Check sheet for the modelled part. Datum: model origin and axes. Units: mm. Round coordinates to 2 decimals unless told otherwise and drop trailing zeros. Write each loop counter-clockwise with the first axis right and the second up, starting at its lowest first coordinate (ties: lowest second). Pieces come first, ordered by that corner, then holes. Notation, with made-up numbers: (-20, -6.5) -> (15, -6.5) arc R29 ccw to (15, 21.5) -> close; hole circle Ø7 at (56.5, -26). An arc over 180 degrees is marked (long way). Put each result on its own line as item: value. Start each with the question number.
from build123d import *

# Parameters (mm, degrees)
F0_R      = 4.6
F1_DEPTH  = 10
F2_R      = 0.95
F4_DEPTH  = 5
F4_FACE_R = 0.95
F3_R      = 2.5


with BuildPart() as f1:
    # F0 (on Top) → F1 (new body)
    with BuildSketch(Plane.XY):
        Circle(F0_R)
    extrude(amount=F1_DEPTH)

    # F2 (on face) → F4 (cut)
    with BuildSketch(Plane(origin=(0, 0, 0), x_dir=(1, 0, 0), z_dir=(0, 0, -1))):
        Circle(F2_R)
    extrude(amount=-F4_DEPTH, mode=Mode.SUBTRACT)

    # F4_face (on face) → F5 section 0
    with BuildSketch(Plane(origin=(0, 0, 5), x_dir=(1, 0, 0), z_dir=(0, 0, -1))):
        Circle(F4_FACE_R)
    # F3 (on face) → F5 section 1
    with BuildSketch(Plane.XY.offset(10)):
        Circle(F3_R)
    loft(mode=Mode.SUBTRACT)


solid = f1.part
1. Section check B-B, the plane z = 8.5. Enter the section's corners in (x, y) (3 decimals), then the cut area to 3 significant figures.
2. Section check C-C, the plane y = -3.25. Enter the section's corners in (x, z), then the cut area to 3 significant figures.
3. Section check A-A, the plane x = 0. Enter the section's corners in (y, z).
4. Section check D-D, the plane x = -3. Enter the section's corners in (y, z), then the cut area to 3 significant figures.
5. Material ranges on L1, parallel to Y at x = 0, z = 3.2; L2, parallel to X at y = -0.75, z = 9.25; L3, parallel to X at y = -0.75, z = 6.5, recorded low to high. Write a range as [from, to].
6. Draft check along Y on faces 1 (the cylindrical face through (-0.95, -0.04, 2.46)), 2 (the cylindrical face through (-3.65, -2.8, 4.93)), 3 (the conical face through (-1.24, 0.95, 6.98)), 4 (the flat face through (2, -2, 10)). Enter one of: released by +Y, released by -Y, zero draft, split by the parting line, or undercut.
7. Gauge pin test, flat ends, axial feed: P1, Ø3, axis at x = -3, z = 7, coming from the +Y side; P2, Ø5, axis at y = 0.5, z = 2, coming from the +X side; P3, Ø2, axis at x = -2.5, z = 8.5, coming from the -Y side. Record the tip position at first contact, or that the pin passes through.
Reply:
1. outline: circle Ø9.2 at (0, 0); hole circle Ø4.07 at (0, 0)
1. area: 53.5 mm2
2. outline: (-3.26, 0) -> (3.26, 0) -> (3.26, 10) -> (-3.26, 10) -> close
2. area: 65.1 mm2
3. outline: (-4.6, 0) -> (-0.95, 0) -> (-0.95, 5) -> (-2.5, 10) -> (-4.6, 10) -> close; (0.95, 0) -> (4.6, 0) -> (4.6, 10) -> (2.5, 10) -> (0.95, 5) -> close
4. outline: (-3.49, 0) -> (3.49, 0) -> (3.49, 10) -> (-3.49, 10) -> close
4. area: 69.7 mm2
5. L1: y = [-4.6, -0.95], [0.95, 4.6]
5. L2: x = [-4.54, -2.14], [2.14, 4.54]
5. L3: x = [-4.54, -1.2], [1.2, 4.54]
6. face 1: undercut
6. face 2: split by the parting line
6. face 3: undercut
6. face 4: zero draft
7. P1: stops at y = 4.35
7. P2: stops at x = 4.6
7. P3: stops at y = -4.35
